For this review, take the finished solid that the model builds, in its own axes (mm). Face numbers are marked on the shaded views. A direction names the side the tool comes from. Give positions to 0.01 mm unless a question says otherwise; leave off trailing zeros. Write each loop counter-clockwise with the first axis right and the second up, starting at its lowest first coordinate (ties: lowest second). Pieces come first, ordered by that corner, then holes.
Q1. For line 1 (X direction, y = -5, z = 3.6); line 2 (Y direction, x = 2, z = 8.25); line 3 (Y direction, x = 6.75, z = 7.5), list the stretches that pass through material, from the lowest coordinate up.
Q2. We need section C-C (y = 7.5). Write out the cut boundary in (x, z).
Q3. Machinability: for the marked faces 1 and 2, which of the approach directions +Z, -Z, +X, -X, +Y, -Y give a long, thin tool a straight path to every point of the face, cutting with its end or side? Answer none if there is none.
Q4. Insertion check: P1, Ø5, axis at x = -2, z = 5, coming from the +Y side; P2, Ø4, axis at x = 4.5, z = 5, coming from the +Y side; P3, Ø1, axis at x = -5.5, z = 6, coming from the -Y side. Each pin has a flat end and moves straight along its axis. Give the tip position at first contact, or say it passes through.
Q5. Mouldability with a two-part tool opening along X and no side actions: class the marked faces 3, 4 and 5 as released by +X, released by -X, zero draft, split by the parting line, or undercut.
Q6. We need section D-D (x = 3). Write out the cut boundary in (y, z).
Q7. We need section A-A (x = -5). Write out the cut boundary in (y, z), then the cut area to 3 significant figures.
Q8. We need section B-B (z = 2). Write out the cut boundary in (x, y).
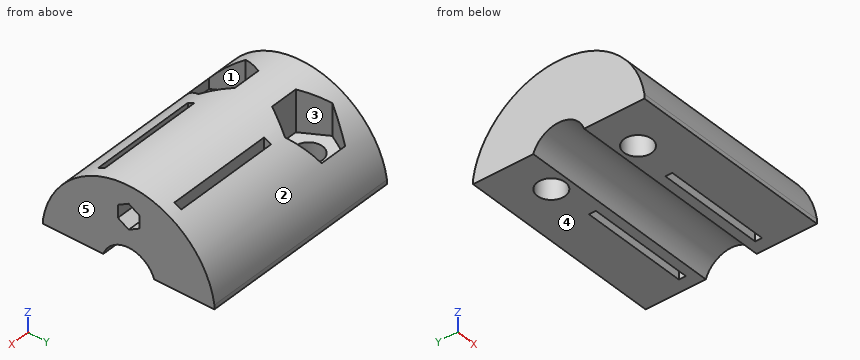
```python
from build123d import *

# Parameters (mm, degrees)
AUFSATZ_LINEAR_AUSTRAGEN1_DEPTH      = 14
AUFSATZ_LINEAR_AUSTRAGEN1_DEPTH_BACK = 10
SKIZZE2_W                            = 12.5
SKIZZE2_H                            = 0.8
SCHNITT_LINEAR_AUSTRAGEN1_DEPTH      = 20.843134833
SCHNITT_LINEAR_START                 = 5
SCHNITT_LINEAR_AUSTRAGEN2_DEPTH      = 15.843134833
SKIZZE4_R                            = 1.6
SCHNITT_LINEAR_AUSTRAGEN3_DEPTH      = 20.843134833
SCHNITT_LINEAR_START_2               = 14
SCHNITT_LINEAR_AUSTRAGEN4_DEPTH      = 10


with BuildPart() as part:
    # Skizze1 → Aufsatz-Linear austragen1 (new, two sides: drawn at the far end of the back side and taken through both)
    with BuildSketch(Plane(origin=(0, 0, 0), x_dir=(0, 0, -1), z_dir=(1, 0, 0)).offset(-AUFSATZ_LINEAR_AUSTRAGEN1_DEPTH_BACK)):
        with BuildLine():
            Line((-1.5, 9.886859967), (-1, 9.886859967))
            Line((-1, 9.886859967), (-1, 2.93428015))
            ThreePointArc((-1, 2.93428015), (-3.1, 0), (-1, -2.93428015))
            Line((-1, -2.93428015), (-1, -9.886859967))
            Line((-1, -9.886859967), (-1.5, -9.886859967))
            ThreePointArc((-1.5, -9.886859967), (-10, 0), (-1.5, 9.886859967))
        make_face()
    extrude(amount=AUFSATZ_LINEAR_AUSTRAGEN1_DEPTH + AUFSATZ_LINEAR_AUSTRAGEN1_DEPTH_BACK)

    # Skizze2 → Schnitt-Linear austragen1 (cut, through all)
    with BuildSketch(Plane.XY):
        with Locations((6.25, 4.4)):
            Rectangle(SKIZZE2_W, SKIZZE2_H)
    schnitt_linear_austragen1 = extrude(amount=SCHNITT_LINEAR_AUSTRAGEN1_DEPTH, mode=Mode.SUBTRACT)

    # Skizze3 → Schnitt-Linear austragen2 (cut, through all)
    with BuildSketch(Plane.XY.offset(SCHNITT_LINEAR_START)):
        Polygon((-3.354551733, 2.15), (-1.709103466, 5), (-3.354551733, 7.85), (-6.645448267, 7.85), (-8.290896534, 5), (-6.645448267, 2.15), align=None)
    schnitt_linear_austragen2 = extrude(amount=SCHNITT_LINEAR_AUSTRAGEN2_DEPTH, mode=Mode.SUBTRACT)

    # Skizze4 → Schnitt-Linear austragen3 (cut, through all)
    with BuildSketch(Plane.XY):
        with Locations(Location((-5, 5, 0), (0, 0, 90))):
            Circle(SKIZZE4_R)
    schnitt_linear_austragen3 = extrude(amount=SCHNITT_LINEAR_AUSTRAGEN3_DEPTH, mode=Mode.SUBTRACT)

    # Spiegeln1: Schnitt-Linear austragen1, Schnitt-Linear austragen2, Schnitt-Linear austragen3 across plane
    add(schnitt_linear_austragen1.mirror(Plane.ZX), mode=Mode.SUBTRACT)
    add(schnitt_linear_austragen2.mirror(Plane.ZX), mode=Mode.SUBTRACT)
    add(schnitt_linear_austragen3.mirror(Plane.ZX), mode=Mode.SUBTRACT)

    # Skizze6 → Schnitt-Linear austragen4 (cut)
    with BuildSketch(Plane(origin=(0, 0, 0), x_dir=(0, 0, -1), z_dir=(1, 0, 0)).offset(SCHNITT_LINEAR_START_2)):
        Polygon((-5.828312164, 1.25), (-7.271687836, 1.25), (-7.993375673, 0), (-7.271687836, -1.25), (-5.828312164, -1.25), (-5.106624327, 0), align=None)
    extrude(amount=-SCHNITT_LINEAR_AUSTRAGEN4_DEPTH, mode=Mode.SUBTRACT)


solid = part.part
```
Computed:
1. line 1: x = -10 to -6.6, -3.4 to 14
1. line 2: y = -5.65 to -4.8, -4 to 4, 4.8 to 5.65
1. line 3: y = -6.61 to -4.8, -4 to -0.85, 0.85 to 4, 4.8 to 6.61
2. outline: (-10, 1) - (14, 1) - (14, 6.61) - (-3.15, 6.61) - (-3.15, 5) - (-6.85, 5) - (-6.85, 6.61) - (-10, 6.61) - close
3. face 1: +Z
3. face 2: +Z, +X, -X
4. P1: stops at y = 9.68
4. P2: stops at y = 9.54
4. P3: stops at y = -8.35
5. face 3: undercut
5. face 4: zero draft
5. face 5: released by +X
6. outline: (-9.89, 1) - (-4.8, 1) - (-4.8, 8.77) arc R10 ccw to (-9.89, 1.5) - close; (-4, 1) - (-2.93, 1) arc R3.1 cw to (2.93, 1) - (4, 1) - (4, 9.17) arc R10 ccw to (-4, 9.17) - close; (4.8, 1) - (9.89, 1) - (9.89, 1.5) arc R10 ccw to (4.8, 8.77) - close
7. outline: (-9.89, 1) - (-6.6, 1) - (-6.6, 5) - (-7.85, 5) - (-7.85, 6.19) arc R10 ccw to (-9.89, 1.5) - close; (-3.4, 1) - (-2.93, 1) arc R3.1 cw to (2.93, 1) - (3.4, 1) - (3.4, 5) - (2.15, 5) - (2.15, 9.77) arc R10 ccw to (-2.15, 9.77) - (-2.15, 5) - (-3.4, 5) - close; (6.6, 1) - (9.89, 1) - (9.89, 1.5) arc R10 ccw to (7.85, 6.19) - (7.85, 5) - (6.6, 5) - close
7. area: 63.2 mm2
8. outline: (-10, -9.8) - (14, -9.8) - (14, -2.37) - (-10, -2.37) - close; (-10, 2.37) - (14, 2.37) - (14, 9.8) - (-10, 9.8) - close; hole circle Ø3.2 at (-5, -5); hole circle Ø3.2 at (-5, 5); hole (0, -4.8) - (12.5, -4.8) - (12.5, -4) - (0, -4) - close; hole (0, 4) - (12.5, 4) - (12.5, 4.8) - (0, 4.8) - close
